Source: CAD feature listing. Evaluate the final solid. Frame: model axes, mm. A direction names the side the tool comes from. Give positions to 0.01 mm unless a question says otherwise; leave off trailing zeros. Loops run counter-clockwise (first coordinate to the right, second up) from the corner with the lowest first, then second, coordinate; pieces in that order, holes last. Notation, with made-up numbers: M 89,74 L 141,74 A19 ccw 141,105 Z; hole C 21.25,-36 d9. An arc over 180 degrees is marked long. Put each result on its own line as item: value. Start each with the question number.
```python
from build123d import *

# Parameters (mm, degrees)
PLATE_MAIN_SKETCH_R                          = 11
PLATE_MAIN_SKETCH_R_2                        = 3
EXTRUDE_PLATE_MAIN_DEPTH                     = 7
CORNER_FILLETS_R                             = 2
M3X0_5_TAPPED_HOLES_AT_2_COUNT               = 2
M3X0_5_TAPPED_HOLES_AT_2_PITCH               = 27.5
M3X0_5_TAPPED_HOLES_AT_3_COUNT               = 2
M3X0_5_TAPPED_HOLES_AT_3_PITCH               = 58.823889705
M3X0_5_TAPPED_HOLES_AT_4_COUNT               = 2
M3X0_5_TAPPED_HOLES_AT_4_PITCH               = 66.206117542
M3X0_5_TAPPED_HOLES_AT_5_COUNT               = 2
M3X0_5_TAPPED_HOLES_AT_5_PITCH               = 83.20606949
M3X0_5_TAPPED_HOLES_AT_6_COUNT               = 2
M3X0_5_TAPPED_HOLES_AT_6_PITCH               = 101.307699609
M3X0_5_TAPPED_HOLES_AT_7_COUNT               = 2
M3X0_5_TAPPED_HOLES_AT_7_PITCH               = 120.013540903
M3X0_5_TAPPED_HOLES_AT_8_COUNT               = 2
M3X0_5_TAPPED_HOLES_AT_8_PITCH               = 114.242067558
M3X0_5_TAPPED_HOLES_AT_9_COUNT               = 2
M3X0_5_TAPPED_HOLES_AT_9_PITCH               = 94.399417371
M3X0_5_TAPPED_HOLES_AT_10_COUNT              = 2
M3X0_5_TAPPED_HOLES_AT_10_PITCH              = 74.640806534
M3X0_5_TAPPED_HOLES_AT_11_COUNT              = 2
M3X0_5_TAPPED_HOLES_AT_11_PITCH              = 55.056788864
M3X0_5_TAPPED_HOLES_AT_12_COUNT              = 2
M3X0_5_TAPPED_HOLES_AT_12_PITCH              = 52
M3_COUNTER_BORES_AT_2_COUNT                  = 2
M3_COUNTER_BORES_AT_2_PITCH                  = 31
M3_COUNTER_BORES_AT_3_COUNT                  = 2
M3_COUNTER_BORES_AT_3_PITCH                  = 43.840620434
M3_COUNTER_BORES_AT_4_COUNT                  = 2
M3_COUNTER_BORES_AT_4_PITCH                  = 31
M3_COUNTER_BORES_AT_5_COUNT                  = 2
M3_COUNTER_BORES_AT_5_PITCH                  = 42.172265768
M3_COUNTER_BORES_AT_6_COUNT                  = 2
M3_COUNTER_BORES_AT_6_PITCH                  = 56.608303278
M3_COUNTER_BORES_AT_7_COUNT                  = 2
M3_COUNTER_BORES_AT_7_PITCH                  = 70.86959856
M3_COUNTER_BORES_AT_8_COUNT                  = 2
M3_COUNTER_BORES_AT_8_PITCH                  = 59.970826241
M3_COUNTER_BORES_AT_9_COUNT                  = 2
M3_COUNTER_BORES_AT_9_PITCH                  = 101.688249075
M3_COUNTER_BORES_AT_10_COUNT                 = 2
M3_COUNTER_BORES_AT_10_PITCH                 = 111.581808553
M5X0_8_TAPPED_HOLE1_D                        = 4.2
CUT_RECESS_DEPTH                             = 1
LEFT_Z_AXIS_SENSORS_M3X0_5_TAPPED_HO_2_COUNT = 2
LEFT_Z_AXIS_SENSORS_M3X0_5_TAPPED_HO_2_PITCH = 19.7


with BuildPart() as part:
    # Plate Main Sketch → Extrude Plate Main (new body)
    with BuildSketch(Plane(origin=(-158.085545862, 0, 24.679095537), x_dir=(-1, 0, 0), z_dir=(0, 1, 0))):
        with BuildLine():
            Line((-178.585545862, -24.679095537), (-137.585545862, -24.679095537))
            Line((-137.585545862, -24.679095537), (-137.585545862, -12.679095537))
            ThreePointArc((-137.585545862, -12.679095537), (-136.121079768, -9.143561631), (-132.585545862, -7.679095537))
            Line((-132.585545862, -7.679095537), (-129.585545862, -7.679095537))
            Line((-129.585545862, -7.679095537), (-129.585545862, 54.820904463))
            ThreePointArc((-129.585545862, 54.820904463), (-128.853312815, 56.588671416), (-127.085545862, 57.320904463))
            Line((-127.085545862, 57.320904463), (-127.085545862, 83.320904463))
            ThreePointArc((-127.085545862, 83.320904463), (-128.853312815, 84.05313751), (-129.585545862, 85.820904463))
            Line((-129.585545862, 85.820904463), (-129.585545862, 101.320904463))
            Line((-129.585545862, 101.320904463), (-186.585545862, 101.320904463))
            Line((-186.585545862, 101.320904463), (-186.585545862, 85.820904463))
            ThreePointArc((-186.585545862, 85.820904463), (-187.317778909, 84.05313751), (-189.085545862, 83.320904463))
            Line((-189.085545862, 83.320904463), (-189.085545862, 57.320904463))
            ThreePointArc((-189.085545862, 57.320904463), (-187.317778909, 56.588671416), (-186.585545862, 54.820904463))
            Line((-186.585545862, 54.820904463), (-186.585545862, -7.679095537))
            Line((-186.585545862, -7.679095537), (-183.585545862, -7.679095537))
            ThreePointArc((-183.585545862, -7.679095537), (-180.050011956, -9.143561631), (-178.585545862, -12.679095537))
            Line((-178.585545862, -12.679095537), (-178.585545862, -24.679095537))
        make_face()
        with Locations(Location((-158.085545862, 80.320904463, 0), (0, 0, 90))):
            Circle(PLATE_MAIN_SKETCH_R, mode=Mode.SUBTRACT)
        with Locations(Location((-145.585545862, 33.320904463, 0), (0, 0, 90))):
            Circle(PLATE_MAIN_SKETCH_R_2, mode=Mode.SUBTRACT)
        with Locations(Location((-170.585545862, 33.320904463, 0), (0, 0, 270))):
            Circle(PLATE_MAIN_SKETCH_R_2, mode=Mode.SUBTRACT)
    extrude(amount=EXTRUDE_PLATE_MAIN_DEPTH)

    # Corner Fillets
    corner_fillets_edges = [part.edges().sort_by_distance(p)[0] for p in [
        (28.5, 3.5, 126),
        (-28.5, 3.5, 126),
        (-28.5, 3.5, 17),
        (-20.5, 3.5, 0),
        (20.5, 3.5, 0),
        (28.5, 3.5, 17),
    ]]
    fillet(corner_fillets_edges, radius=CORNER_FILLETS_R)

    # Sketch13 → M3x0.5 Tapped Holes (revolve, cut)
    with BuildSketch(Plane(origin=(26, 0, 121.5), x_dir=(0, 0, -1), z_dir=(1, 0, 0))):
        Polygon((0, 0), (0, 7), (1.725, 7), (1.25, 6.525), (1.25, 0), align=None)
    m3x0_5_tapped_holes = revolve(axis=Axis((26, -6.35, 121.5), (0, 1, 0)), mode=Mode.SUBTRACT)

    # M3x0.5 Tapped Holes at 2: M3x0.5 Tapped Holes ×2
    with Locations(*[(0, 0, -i * M3X0_5_TAPPED_HOLES_AT_2_PITCH) for i in range(1, M3X0_5_TAPPED_HOLES_AT_2_COUNT)]):
        add(m3x0_5_tapped_holes, mode=Mode.SUBTRACT)

    # M3x0.5 Tapped Holes at 3: M3x0.5 Tapped Holes ×2
    with Locations(*[Vector(-0.8839945855497452, 0, -0.46749713658880765) * (i * M3X0_5_TAPPED_HOLES_AT_3_PITCH) for i in range(1, M3X0_5_TAPPED_HOLES_AT_3_COUNT)]):
        add(m3x0_5_tapped_holes, mode=Mode.SUBTRACT)

    # M3x0.5 Tapped Holes at 4: M3x0.5 Tapped Holes ×2
    with Locations(*[Vector(-0.5890694311623529, 0, -0.8080824247996377) * (i * M3X0_5_TAPPED_HOLES_AT_4_PITCH) for i in range(1, M3X0_5_TAPPED_HOLES_AT_4_COUNT)]):
        add(m3x0_5_tapped_holes, mode=Mode.SUBTRACT)

    # M3x0.5 Tapped Holes at 5: M3x0.5 Tapped Holes ×2
    with Locations(*[Vector(-0.46871580689935055, 0, -0.8833490206949294) * (i * M3X0_5_TAPPED_HOLES_AT_5_PITCH) for i in range(1, M3X0_5_TAPPED_HOLES_AT_5_COUNT)]):
        add(m3x0_5_tapped_holes, mode=Mode.SUBTRACT)

    # M3x0.5 Tapped Holes at 6: M3x0.5 Tapped Holes ×2
    with Locations(*[Vector(-0.38496580369162126, 0, -0.9229308370555532) * (i * M3X0_5_TAPPED_HOLES_AT_6_PITCH) for i in range(1, M3X0_5_TAPPED_HOLES_AT_6_COUNT)]):
        add(m3x0_5_tapped_holes, mode=Mode.SUBTRACT)

    # M3x0.5 Tapped Holes at 7: M3x0.5 Tapped Holes ×2
    with Locations(*[Vector(-0.32496333085967716, 0, -0.9457266167326497) * (i * M3X0_5_TAPPED_HOLES_AT_7_PITCH) for i in range(1, M3X0_5_TAPPED_HOLES_AT_7_COUNT)]):
        add(m3x0_5_tapped_holes, mode=Mode.SUBTRACT)

    # M3x0.5 Tapped Holes at 8: M3x0.5 Tapped Holes ×2
    with Locations(*[Vector(-0.113793458730633, 0, -0.993504428148219) * (i * M3X0_5_TAPPED_HOLES_AT_8_PITCH) for i in range(1, M3X0_5_TAPPED_HOLES_AT_8_COUNT)]):
        add(m3x0_5_tapped_holes, mode=Mode.SUBTRACT)

    # M3x0.5 Tapped Holes at 9: M3x0.5 Tapped Holes ×2
    with Locations(*[Vector(-0.13771271435815216, 0, -0.9904722148067102) * (i * M3X0_5_TAPPED_HOLES_AT_9_PITCH) for i in range(1, M3X0_5_TAPPED_HOLES_AT_9_COUNT)]):
        add(m3x0_5_tapped_holes, mode=Mode.SUBTRACT)

    # M3x0.5 Tapped Holes at 10: M3x0.5 Tapped Holes ×2
    with Locations(*[Vector(-0.17416746420246676, 0, -0.9847160476062541) * (i * M3X0_5_TAPPED_HOLES_AT_10_PITCH) for i in range(1, M3X0_5_TAPPED_HOLES_AT_10_COUNT)]):
        add(m3x0_5_tapped_holes, mode=Mode.SUBTRACT)

    # M3x0.5 Tapped Holes at 11: M3x0.5 Tapped Holes ×2
    with Locations(*[Vector(-0.23611983677697992, 0, -0.9717239436591096) * (i * M3X0_5_TAPPED_HOLES_AT_11_PITCH) for i in range(1, M3X0_5_TAPPED_HOLES_AT_11_COUNT)]):
        add(m3x0_5_tapped_holes, mode=Mode.SUBTRACT)

    # M3x0.5 Tapped Holes at 12: M3x0.5 Tapped Holes ×2
    with Locations(*[(-i * M3X0_5_TAPPED_HOLES_AT_12_PITCH, 0, 0) for i in range(1, M3X0_5_TAPPED_HOLES_AT_12_COUNT)]):
        add(m3x0_5_tapped_holes, mode=Mode.SUBTRACT)

    # Sketch5 → M3 Counter Bores (revolve, cut)
    with BuildSketch(Plane(origin=(-15.5, 0, 120.5), x_dir=(0, 0, -1), z_dir=(1, 0, 0))):
        Polygon((0, 0), (0, 7), (1.725, 7), (1.7, 6.975), (1.7, 4.5), (3, 4.5), (3, 0), align=None)
    m3_counter_bores = revolve(axis=Axis((-15.5, -6.35, 120.5), (0, 1, 0)), mode=Mode.SUBTRACT)

    # M3 Counter Bores at 2: M3 Counter Bores ×2
    with Locations(*[(i * M3_COUNTER_BORES_AT_2_PITCH, 0, 0) for i in range(1, M3_COUNTER_BORES_AT_2_COUNT)]):
        add(m3_counter_bores, mode=Mode.SUBTRACT)

    # M3 Counter Bores at 3: M3 Counter Bores ×2
    with Locations(*[Vector(0.7071067811865479, 0, -0.7071067811865472) * (i * M3_COUNTER_BORES_AT_3_PITCH) for i in range(1, M3_COUNTER_BORES_AT_3_COUNT)]):
        add(m3_counter_bores, mode=Mode.SUBTRACT)

    # M3 Counter Bores at 4: M3 Counter Bores ×2
    with Locations(*[(0, 0, -i * M3_COUNTER_BORES_AT_4_PITCH) for i in range(1, M3_COUNTER_BORES_AT_4_COUNT)]):
        add(m3_counter_bores, mode=Mode.SUBTRACT)

    # M3 Counter Bores at 5: M3 Counter Bores ×2
    with Locations(*[Vector(-0.1778419978967634, 0, -0.9840590550287557) * (i * M3_COUNTER_BORES_AT_5_PITCH) for i in range(1, M3_COUNTER_BORES_AT_5_COUNT)]):
        add(m3_counter_bores, mode=Mode.SUBTRACT)

    # M3 Counter Bores at 6: M3 Counter Bores ×2
    with Locations(*[Vector(0.6801122409730789, 0, -0.7331080000099417) * (i * M3_COUNTER_BORES_AT_6_PITCH) for i in range(1, M3_COUNTER_BORES_AT_6_COUNT)]):
        add(m3_counter_bores, mode=Mode.SUBTRACT)

    # M3 Counter Bores at 7: M3 Counter Bores ×2
    with Locations(*[Vector(0.5432512781572745, 0, -0.8395701571521512) * (i * M3_COUNTER_BORES_AT_7_PITCH) for i in range(1, M3_COUNTER_BORES_AT_7_COUNT)]):
        add(m3_counter_bores, mode=Mode.SUBTRACT)

    # M3 Counter Bores at 8: M3 Counter Bores ×2
    with Locations(*[Vector(-0.12506080823181873, 0, -0.9921490786390946) * (i * M3_COUNTER_BORES_AT_8_PITCH) for i in range(1, M3_COUNTER_BORES_AT_8_COUNT)]):
        add(m3_counter_bores, mode=Mode.SUBTRACT)

    # M3 Counter Bores at 9: M3 Counter Bores ×2
    with Locations(*[Vector(0.15242665834989907, 0, -0.9883147847848291) * (i * M3_COUNTER_BORES_AT_9_PITCH) for i in range(1, M3_COUNTER_BORES_AT_9_COUNT)]):
        add(m3_counter_bores, mode=Mode.SUBTRACT)

    # M3 Counter Bores at 10: M3 Counter Bores ×2
    with Locations(*[Vector(0.13891153227375555, 0, -0.9903047945967733) * (i * M3_COUNTER_BORES_AT_10_PITCH) for i in range(1, M3_COUNTER_BORES_AT_10_COUNT)]):
        add(m3_counter_bores, mode=Mode.SUBTRACT)

    # M5x0.8 Tapped Hole1 (through all)
    with Locations(Plane(origin=(0, 0, 0), x_dir=(-1, 0, 0), z_dir=(0, -1, 0))):
        with Locations((0, -79.5)):
            Hole(M5X0_8_TAPPED_HOLE1_D / 2)

    # Reccess Sketch → Cut Recess (cut)
    with BuildSketch(Plane(origin=(0, 0, 0), x_dir=(1, 0, 0), z_dir=(0, 1, 0))):
        with BuildLine():
            Line((-8.25, 0), (-8.25, -81))
            ThreePointArc((-8.25, -81), (-9.128679656, -83.121320344), (-11.25, -84))
            Line((-11.25, -84), (-31, -84))
            Line((-31, -84), (-31, 0))
            Line((-31, 0), (-8.25, 0))
        make_face()
        with BuildLine():
            Line((31, 0), (8.25, 0))
            Line((8.25, 0), (8.25, -81))
            ThreePointArc((8.25, -81), (9.128679656, -83.121320344), (11.25, -84))
            Line((11.25, -84), (31, -84))
            Line((31, -84), (31, 0))
        make_face()
    extrude(amount=CUT_RECESS_DEPTH, mode=Mode.SUBTRACT)

    # Sketch17 → Left Z-Axis Sensors M3x0.5 Tapped Holes (revolve, cut)
    with BuildSketch(Plane(origin=(-31, 3.5, 85.15), x_dir=(0, 0, 1), z_dir=(0, 1, 0))):
        Polygon((0, 0), (0, 10.751075774), (1.25, 10), (1.25, 0), align=None)
    left_z_axis_sensors_m3x0_5_tapped_holes = revolve(axis=Axis((-37.35, 3.5, 85.15), (1, 0, 0)), mode=Mode.SUBTRACT)

    # Left Z-Axis Sensors M3x0.5 Tapped Ho 2: Left Z-Axis Sensors M3x0.5 Tapped Holes ×2
    with Locations(*[(0, 0, i * LEFT_Z_AXIS_SENSORS_M3X0_5_TAPPED_HO_2_PITCH) for i in range(1, LEFT_Z_AXIS_SENSORS_M3X0_5_TAPPED_HO_2_COUNT)]):
        add(left_z_axis_sensors_m3x0_5_tapped_holes, mode=Mode.SUBTRACT)

    # Right Z-Axis Sensor Holes Mirror: Left Z-Axis Sensors M3x0.5 Tapped Holes across plane
    add(left_z_axis_sensors_m3x0_5_tapped_holes.mirror(Plane(origin=(0, 0, 0), x_dir=(0, 0, 1), z_dir=(1, 0, 0))), mode=Mode.SUBTRACT)

    # Right Z-Axis Sensor Holes Mirror copy 1 → Right Z-Axis Sensor Holes Mirror cop 2 (revolve, cut)
    with BuildSketch(Plane(origin=(31, 3.5, 104.85), x_dir=(0, 0, 1), z_dir=(0, 1, 0))):
        Polygon((0, 0), (0, -10.751075774), (1.25, -10), (1.25, 0), align=None)
    revolve(axis=Axis((37.35, 3.5, 104.85), (1, 0, 0)), mode=Mode.SUBTRACT)


solid = part.part
```
1. Section B-B, the plane x = 6. Output: boundary loops of the cut face in (y, z).
2. Set-up query: faces 1 (the face through (28.5, 3, 117)), 2 (the face through (-26.07, 3.12, 106.04)), 3 (the face through (20.5, 4, 7)), 4 (the face through (-28.5, 4, 49)). Return all of +Z, -Z, +X, -X, +Y, -Y with unobstructed straight access to the full face (end or side cutting, diameter ignored); none if empty.
3. Pull-direction query (Y, two-part tool) for faces 5 (the face through (2, 4.5, 10)), 6 (the face through (26.07, 3.12, 106.04)), 7 (the face through (26.479, 3.217, 92.845)); classes: released by +Y, released by -Y, zero draft, split by the parting line, or undercut.
4. Contact query for flat-ended pins moving along their axis: pin 1 (7 mm diameter, centred on x = 22, z = 40.5, fed in from -Y); pin 2 (3.5 mm diameter, centred on x = -15.5, z = 89.5, fed in from -Y); pin 3 (0.5 mm diameter, centred on y = 0.5, z = 35, fed in from -X). Output: stop coordinate, or through.
5. Section A-A, the plane z = 48. Output: boundary loops of the cut face in (x, y) (3 decimals).
6. Ray query, line 1 (X direction, y = 5.3, z = 68); line 2 (X direction, y = 1.5, z = 105); line 3 (X direction, y = 1.1, z = 120.5). Return the intervals inside material, ascending.
Results found:
1. outline: M 0,0 L 7,0 L 7,95.78 L 0,95.78 Z; M 0,114.22 L 7,114.22 L 7,126 L 0,126 Z
2. face 1: +Z, +X, +Y, -Y
2. face 2: -X
2. face 3: -Z, +X, +Y, -Y
2. face 4: -Z, -X, +Y, -Y
3. face 5: released by -Y
3. face 6: undercut
3. face 7: zero draft
4. pin 1: y = 1
4. pin 2: y = 4.5
4. pin 3: x = -8.25
5. outline: M -28.5,1 L -14.25,1 L -14.25,6.525 L -14.725,7 L -28.5,7 Z; M -11.75,1 L -8.25,1 L -8.25,0 L 8.25,0 L 8.25,1 L 11.75,1 L 11.75,6.525 L 11.275,7 L -11.275,7 L -11.75,6.525 Z; M 14.25,1 L 28.5,1 L 28.5,7 L 14.725,7 L 14.25,6.525 Z
6. line 1: -28.5 to -14.25, -11.75 to 11.75, 14.25 to 28.5
6. line 2: -31 to -11, 11 to 31
6. line 3: -28.5 to -26.75, -25.25 to -18.5, -12.5 to 12.5, 18.5 to 25.25, 26.75 to 28.5
